from build123d import *

# Parameters (mm, degrees)
CYLINDER003_R     = 2
CYLINDER003_DEPTH = 10
CYLINDER002_R     = 2
CYLINDER002_DEPTH = 10
BOX003_W          = 5
BOX003_H          = 100
BOX003_DEPTH      = 2
BOX_W             = 10
BOX_H             = 100
BOX_DEPTH         = 20
FILLET_R          = 4
FILLET001_R       = 4


with BuildPart() as m3threadhole001:
    # Cylinder003 → Cylinder003 (new body)
    with BuildSketch(Plane(origin=(20, 105, 4), x_dir=(1, 0, 0), z_dir=(0, -1, 0))):
        Circle(CYLINDER003_R)
    extrude(amount=CYLINDER003_DEPTH)


with BuildPart() as fusion001:
    # Cylinder002 → Cylinder002 (new body)
    with BuildSketch(Plane(origin=(20, 15, 4), x_dir=(1, 0, 0), z_dir=(0, -1, 0))):
        Circle(CYLINDER002_R)
    extrude(amount=CYLINDER002_DEPTH)

    # Fusion001: union M3ThreadHole001
    add(m3threadhole001.part)


with BuildPart() as clampstep:
    # Box003 → Box003 (new body)
    with BuildSketch(Plane(origin=(20, 5, 18), x_dir=(1, 0, 0), z_dir=(0, 0, 1))):
        with Locations((2.5, 50)):
            Rectangle(BOX003_W, BOX003_H)
    extrude(amount=BOX003_DEPTH)


with BuildPart() as obj1:
    # Box → Box (new body)
    with BuildSketch(Plane(origin=(15, 5, 0), x_dir=(1, 0, 0), z_dir=(0, 0, 1))):
        with Locations((5, 50)):
            Rectangle(BOX_W, BOX_H)
    extrude(amount=BOX_DEPTH)

    # Cut002: cut ClampStep
    add(clampstep.part, mode=Mode.SUBTRACT)

    # Cut003: cut Fusion001
    add(fusion001.part, mode=Mode.SUBTRACT)

    # Fillet
    fillet_edges = [obj1.edges().sort_by_distance(p)[0] for p in [
        (15, 55, 0),
    ]]
    fillet(fillet_edges, radius=FILLET_R)

    # Fillet001
    fillet001_edges = [obj1.edges().sort_by_distance(p)[0] for p in [
        (25, 55, 0),
    ]]
    fillet(fillet001_edges, radius=FILLET001_R)


solid = obj1.part
Geometry: final body of the model. Coordinates: model frame, mm. A direction names the side the tool comes from. Round coordinates to 2 decimals unless told otherwise and drop trailing zeros. Order: outer loops, then holes, each group sorted by start corner. A loop starts at its lowest first (then second) coordinate and runs counter-clockwise, first axis right, second up.
Q1. Section D-D, the plane x = 16. Output: boundary loops of the cut face in (y, z), and give its area (3 significant figures).
Result sheet:
outline: (5, 1.35) - (105, 1.35) - (105, 20) - (5, 20) - close
area: 1,860 mm2
Q2. Mould query, pull axis Z, two halves, no side actions, for faces 4 (the face through (20, 15, 4)), 5 (the face through (25, 54, 11)), 6 (the face through (16.141, 55.7, 1.203)). Classes: released by +Z, released by -Z, zero draft, split by the parting line, or undercut.
Result sheet:
face 4: undercut
face 5: zero draft
face 6: released by -Z
Q3. Section C-C, the plane z = 3. Output: boundary loops of the cut face in (x, y).
Result sheet:
outline: (15.13, 5) - (18.27, 5) - (18.27, 15) - (21.73, 15) - (21.73, 5) - (24.87, 5) - (24.87, 105) - (21.73, 105) - (21.73, 95) - (18.27, 95) - (18.27, 105) - (15.13, 105) - close
Q4. Section B-B, the plane y = 88. Output: boundary loops of the cut face in (x, z), and give its area (3 significant figures).
Result sheet:
outline: (15, 4) arc R4 ccw to (19, 0) - (21, 0) arc R4 ccw to (25, 4) - (25, 18) - (20, 18) - (20, 20) - (15, 20) - close
area: 183 mm2
Q5. Access query for faces 1 (the face through (20, 54, 19)), 2 (the face through (18.4, 10.1, 2.8)), 3 (the face through (20, 95, 4)). Directions: +Z, -Z, +X, -X, +Y, -Y. A direction counts if a zero-diameter tool reaches every point of the face in a straight line with its end or side. Return the directions, or none.
Result sheet:
face 1: +Z, +X, +Y, -Y
face 2: -Y
face 3: +Y
Q6. Section A-A, the plane y = 11. Output: boundary loops of the cut face in (x, z), and give its area (3 significant figures).
Result sheet:
outline: (15, 4) arc R4 ccw to (19, 0) - (21, 0) arc R4 ccw to (25, 4) - (25, 18) - (20, 18) - (20, 20) - (15, 20) - close; hole circle Ø4 at (20, 4)
area: 171 mm2
Q7. Pin query (flat end, axial travel): pin 1 (4.5 mm diameter, centred on x = 20, z = 4, fed in from -Y); pin 2 (4 mm diameter, centred on x = 16.5, y = 49, fed in from -Z); pin 3 (1 mm diameter, centred on y = 68, z = 19.5, fed in from +X); pin 4 (2.5 mm diameter, centred on x = 20, z = 4, fed in from +Y). Return the tip coordinate at first contact, or that it passes through.
Result sheet:
pin 1: stops at y = 5
pin 2: stops at z = 0.03
pin 3: stops at x = 20
pin 4: stops at y = 95
Q8. Material intervals for probe 1 along Y at (x, z) = (18.5, 5); probe 2 along Z at (x, y) = (20.75, 96.5); probe 3 along Z at (x, y) = (20.5, 71.5), sorted ascending.
Result sheet:
probe 1: y = 15 to 95
probe 2: z = 0 to 2.15, 5.85 to 18
probe 3: z = 0 to 18
